Can you work these out from the drawing? Everything is in mm from the part's minimum corner. A direction names the side the tool comes from. Round coordinates to 2 decimals unless told otherwise and drop trailing zeros. Order: outer loops, then holes, each group sorted by start corner. A loop starts at its lowest first (then second) coordinate and runs counter-clockwise, first axis right, second up. Notation, with made-up numbers: M -32.75,61 L -2.75,61 A29 ccw -2.75,85 Z; hole C 61.5,-1 d10. An arc over 180 degrees is marked long. Write item = value, one per line. Start each with the question number.
Item 1: I want a section at A-A, the plane y = 7.5. List the corners of the cut face in (x, z) for me, plus the area to 3 significant figures.
Item 2: Please list where these lines run through material, in increasing order: L1, parallel to X at y = 2.5, z = 10; L2, parallel to X at y = 3.5, z = 8.25; L3, parallel to Y at x = 9.25, z = 6.5.
Item 3: We'd pull the mould along Z, two halves only. Please class the marked faces 1, 2 and 3: pulls with the +Z half, pulls with the -Z half, needs draft (parallel to the pull), parting line crosses it, or undercut.
Item 4: For the marked faces 4 and 5, which set-ups out of +Z, -Z, +X, -X, +Y, -Y let a thin tool reach every point of the face, with its end or its side?
Item 5: I want a section at C-C, the plane x = 1.75. List the corners of the cut face in (y, z) for me, plus the area to 3 significant figures.
Item 6: I'm going to push flat-ended pins straight in: P1, Ø1, axis at y = 12, z = 9.5, coming from the +X side; P2, Ø8, axis at x = 16.5, y = 6.5, coming from the +Z side; P3, Ø6, axis at x = 8.5, y = 7, coming from the -Z side. Where does each tip first touch, or does it pass through?
Item 7: I want a section at D-D, the plane x = 8.75. List the corners of the cut face in (y, z) for me.
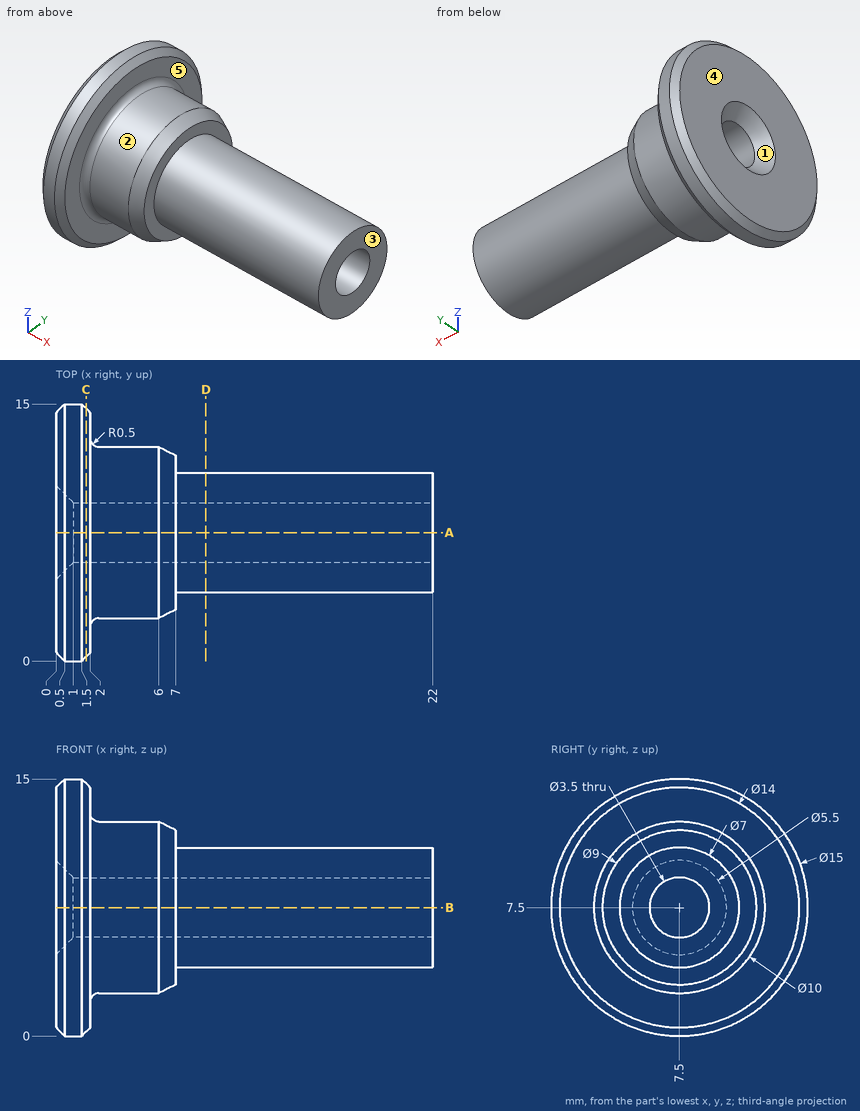
Filled in:
q1.outline = M 0,0.5 L 0.5,0 L 1.5,0 L 2,0.5 L 2,2 A0.5 cw 2.5,2.5 L 6,2.5 L 7,3 L 7,4 L 22,4 L 22,5.75 L 1,5.75 L 0,4.75 Z; M 0,10.25 L 1,9.25 L 22,9.25 L 22,11 L 7,11 L 7,12 L 6,12.5 L 2.5,12.5 A0.5 cw 2,13 L 2,14.5 L 1.5,15 L 0.5,15 L 0,14.5 Z
q1.area = 106 mm^2
q2.L1 = 0 to 2
q2.L2 = 0 to 7
q2.L3 = 4.15 to 6.06, 8.94 to 10.85
q3.face_1 = undercut
q3.face_2 = parting line crosses it
q3.face_3 = needs draft
q4.face_4 = +Z, -Z, -X, +Y, -Y
q4.face_5 = +X
q5.outline = C 7.5,7.5 d14.5; hole C 7.5,7.5 d3.5
q5.area = 156 mm^2
q6.P1 = 7
q6.P2 = 11
q6.P3 = 2.5
q7.outline = C 7.5,7.5 d7; hole C 7.5,7.5 d3.5
